Read the model definition and answer for the solid it produces. Units are mm, in the model's axes. Coordinates: 2 decimals unless noted, no trailing zeros. Write each loop counter-clockwise with the first axis right and the second up, starting at its lowest first coordinate (ties: lowest second). Pieces come first, ordered by that corner, then holes.
(1) The part is cut by section B-B, the plane z = 2.25. State how many separate pieces and enclosed holes the cut face has, and give its area (3 significant figures).
(2) The part is cut by section D-D, the plane y = 129.5. Determine the outline of the cut face in (x, z), and give its area (3 significant figures).
(3) The part is cut by section C-C, the plane x = -114.5. Determine the outline of the cut face in (y, z), and give its area (3 significant figures).
(4) Straight lines are drawn through the part: line 1 along Y through (x, z) = (114.3, 3.75); line 2 along Y through (x, z) = (-25.4, 2.7); line 3 along X through (y, z) = (171, 5.15). For each, find the intervals that lie inside material, in ascending order.
(5) The part is cut by section A-A, the plane y = 171. Determine the outline of the cut face in (x, z).
(6) Given pin 1 (2 mm diameter, centred on y = 130, z = 3, fed in from +X); pin 2 (1 mm diameter, centred on x = -125, y = 67.5, fed in from -Z), each flat-ended and moving along its own axis, determine where each tip first touches the part or whether it passes through.
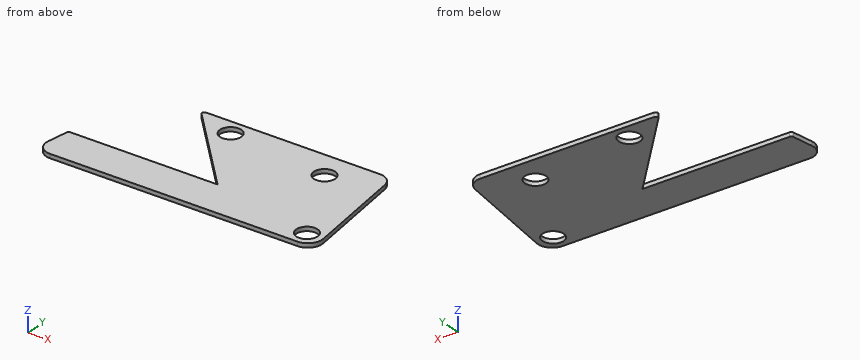
Autodesk Inventor part; units mm, degrees
ref_plane "YZ Plane" through (0, 0, 0) normal (1, 0, 0) x (0, 1, 0)
ref_plane "XZ Plane" through (0, 0, 0) normal (0, 1, 0) x (-1, 0, 0)
ref_plane "XY Plane" through (0, 0, 0) normal (0, 0, 1) x (1, 0, 0)
sketch "Sketch1" plane through (0, 0, 0) normal (0, 0, 1) x (1, 0, 0)
  line L0 (-177.5744, 25.4) -> (-152.1744, 203.2)
  line L1 (-152.1744, 203.2) -> (178.0256, 203.2)
  line L2 (178.0256, 203.2) -> (203.4256, 25.4)
  line L3 (203.4256, 25.4) -> (-177.5744, 25.4)
  circle A0 centre (114.3, 165.1) radius 14.2875
  circle A1 centre (-25.4, 180.975) radius 14.2875
  circle A2 centre (177.8, 47.625) radius 14.2875
  circle A3 centre (505.2413, 166.6875) radius 88.9 construction
  line L4 (-713.704, 0) -> (0, 0) construction
  line L5 (0, 0) -> (0, -152.4) construction
  line L6 (0, -152.4) -> (-713.704, -152.4) construction
  line L7 (-713.704, -152.4) -> (-713.704, 0) construction
  circle A4 centre (177.8, 47.625) radius 50.8 construction
  line L8 (0, -152.4) -> (745.4464, -152.4) construction
  dimension "d0" = 28.575
  dimension "d1" = 22.225
  dimension "d2" = 22.225
  dimension "d7" = 177.8
  dimension "d8" = 152.4
  dimension "d9" = 101.6
  dimension "d11" = 177.8
  dimension "d12" = 25.4
  dimension "d13" = 177.8
  dimension "d14" = 22.225
  dimension "d15" = 203.2
  dimension "d16" = 38.1
  dimension "d17" = 63.5
  dimension "d18" = 381
  dimension "d19" = 330.2
extrude "Extrusion1" add sketch "Sketch1" along normal blind 5.588
fillet "Fillet1" radius 19.05 4 edges at (203.4256, 25.4, 2.794) (178.0256, 203.2, 2.794) (-152.1744, 203.2, 2.794) (-177.5744, 25.4, 2.794)
sketch "Sketch2" plane through (0, 0, 5.588) normal (0, 0, 1) x (1, 0, 0)
  line L0 (-154.5109, 186.8441) -> (-174.4681, 47.1441)
  line L1 (-170.014, 78.3223) -> (33.186, 78.3223)
  line L2 (33.186, 78.3223) -> (-82.5653, 203.2)
  line L3 (161.5037, 203.2) -> (-135.6524, 203.2)
  line L4 (-82.5653, 203.2) -> (-152.1744, 203.2)
  line L5 (-152.1744, 203.2) -> (-170.014, 78.3223)
  point P0 (0, 0)
  dimension "d23" = 203.2
extrude "Extrusion2" cut sketch "Sketch2" against normal through all
fillet "Fillet2" radius 3.175 2 edges at (-170.014, 78.3223, 2.794) (-82.5653, 203.2, 2.794)
properties part number "2021 Intake Panels" material "Polycarbonate, Clear"
Computed:
1. separate pieces: 1
1. enclosed holes: 3
1. area: 44,000 mm2
2. outline: (-14.25, 0) - (188.55, 0) - (188.55, 5.59) - (-14.25, 5.59) - close
2. area: 1,130 mm2
3. outline: (25.4, 0) - (78.32, 0) - (78.32, 5.59) - (25.4, 5.59) - close
3. area: 296 mm2
4. line 1: y = 25.4 to 150.81, 179.39 to 203.2
4. line 2: y = 25.4 to 78.32, 141.53 to 166.69, 195.26 to 203.2
4. line 3: x = -52.72 to -35.63, -15.17 to 101.29, 127.31 to 182.63
5. outline: (-52.72, 0) - (-35.63, 0) - (-35.63, 5.59) - (-52.72, 5.59) - close; (-15.17, 0) - (101.29, 0) - (101.29, 5.59) - (-15.17, 5.59) - close; (127.31, 0) - (182.63, 0) - (182.63, 5.59) - (127.31, 5.59) - close
6. pin 1: stops at x = 188.63
6. pin 2: stops at z = 0
